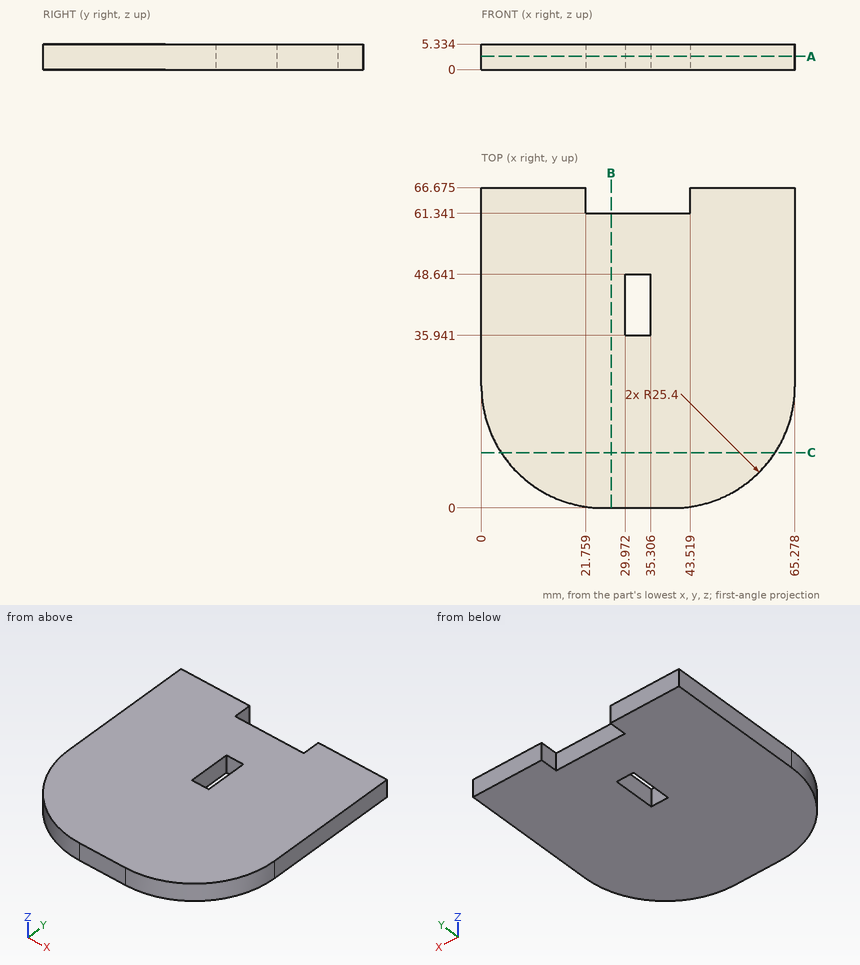
Input: dimensioned drawing with shaded views. Units: mm. Origin: part minimum x, y, z. Give positions to 0.01 mm unless a question says otherwise; leave off trailing zeros. Write each loop counter-clockwise with the first axis right and the second up, starting at its lowest first coordinate (ties: lowest second). Pieces come first, ordered by that corner, then holes. Notation, with made-up numbers: (63, 18) - (84, 18) arc R16 ccw to (84, 28) - close; hole circle Ø6 at (30, 46). An arc over 180 degrees is marked (long way). One line per item, written item: value. Start each with the question number.
Q1. Material intervals for probe 1 along X at (y, z) = (43.5, 0.35); probe 2 along Y at (x, z) = (31.5, 2.95); probe 3 along Y at (x, z) = (38.5, 2.05), sorted ascending. Write a range as from..to.
Q2. Section query B-B, the plane x = 27. Return the cut outline in (y, z).
Q3. First-contact query: pin 1 Ø2 at (y, z) = (18.5, 1) entering from -X (1 decimal); pin 2 Ø2.5 at (x, z) = (33, 3.5) entering from +Y. Flat tips, straight axial feed; report the tip coordinate or a pass-through.
Q4. Section query C-C, the plane y = 11.5. Return the cut outline in (x, z), then the cut area to 3 significant figures.
Q5. Section query A-A, the plane z = 2.75. Return the cut outline in (x, y) (1 decimal).
Answer:
1. probe 1: x = 0..29.97, 35.31..65.28
1. probe 2: y = 0..35.94, 48.64..61.34
1. probe 3: y = 0..61.34
2. outline: (0, 0) - (61.34, 0) - (61.34, 5.33) - (0, 5.33) - close
3. pin 1: stops at x = 0.7
3. pin 2: stops at y = 61.34
4. outline: (4.14, 0) - (61.14, 0) - (61.14, 5.33) - (4.14, 5.33) - close
4. area: 304 mm2
5. outline: (0, 25.4) arc R25.4 ccw to (25.4, 0) - (39.9, 0) arc R25.4 ccw to (65.3, 25.4) - (65.3, 66.7) - (43.5, 66.7) - (43.5, 61.3) - (21.8, 61.3) - (21.8, 66.7) - (0, 66.7) - close; hole (30, 35.9) - (35.3, 35.9) - (35.3, 48.6) - (30, 48.6) - close
